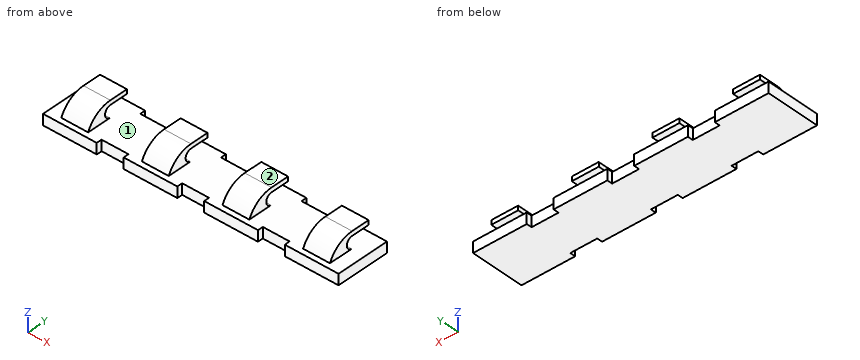
```python
from build123d import *

# Parameters (mm, degrees)
F0_W        = 5
F0_H        = 8
F1_DEPTH    = 2
F2_DEPTH    = 5
F3_T1_DEPTH = 27.9128784748
F3_T3_DEPTH = 27.9128784748
F3_T5_DEPTH = 27.9128784748
F3_T7_DEPTH = 27.9128784748
F5_DEPTH    = 65


# Not quite as in the source:
# - a fillet or chamfer that OpenCascade refuses, or shapes differently, is made with other operations: its cross-section is extruded or revolved along the edge and cut away or added


with BuildPart() as f1:
    # F0 (on Top) → F1 (new body)
    with BuildSketch(Plane.XY):
        Polygon((-17.5, 5), (-27.5, 5), (-27.5, -5), (-17.5, -5), (-17.5, -4), (-17.5, 4), align=None)
        with Locations((-22.5, 0)):
            Rectangle(F0_W, F0_H, mode=Mode.SUBTRACT)
        with Locations((-15, 0)):
            Rectangle(F0_W, F0_H)
        Polygon((-12.5, 5), (-12.5, 4), (-12.5, -4), (-12.5, -5), (-2.5, -5), (-2.5, -4), (-2.5, 4), (-2.5, 5), align=None)
        with Locations((-7.5, 0)):
            Rectangle(F0_W, F0_H, mode=Mode.SUBTRACT)
        Rectangle(F0_W, F0_H)
        Polygon((2.5, 5), (2.5, 4), (2.5, -4), (2.5, -5), (12.5, -5), (12.5, -4), (12.5, 4), (12.5, 5), align=None)
        with Locations((7.5, 0)):
            Rectangle(F0_W, F0_H, mode=Mode.SUBTRACT)
        with Locations((15, 0)):
            Rectangle(F0_W, F0_H)
        Polygon((17.5, 5), (17.5, 4), (17.5, -4), (17.5, -5), (27.5, -5), (27.5, 5), align=None)
        with Locations((22.5, 0)):
            Rectangle(F0_W, F0_H, mode=Mode.SUBTRACT)
    extrude(amount=F1_DEPTH)

    # F0 (on Top) → F2 (join)
    with BuildSketch(Plane.XY):
        with Locations((-22.5, 0)):
            Rectangle(F0_W, F0_H)
        with Locations((-7.5, 0)):
            Rectangle(F0_W, F0_H)
        with Locations((7.5, 0)):
            Rectangle(F0_W, F0_H)
        with Locations((22.5, 0)):
            Rectangle(F0_W, F0_H)
    extrude(amount=F2_DEPTH)

    # F3: fillet of radius 5 on 4 edges, made by hand

    # F3_s2 → F3_t1 (cut)
    with BuildSketch(Plane.YZ.offset(-36.4564392374)):
        with BuildLine():
            ThreePointArc((-4, 2), (-2.1560370926, 4.1833001327), (0.582575695, 5))
            Line((0.582575695, 5), (0.582575695, 5.1))
            Line((0.582575695, 5.1), (-4, 5.1))
            Line((-4, 5.1), (-4.1, 5))
            ThreePointArc((-4.1, 5), (-4.1, 3.5), (-4.0916515139, 2.04))
            Line((-4.0916515139, 2.04), (-4, 2))
        make_face()
    extrude(amount=F3_T1_DEPTH, mode=Mode.SUBTRACT)

    # F3_s4 → F3_t3 (cut)
    with BuildSketch(Plane.YZ.offset(-21.4564392374)):
        with BuildLine():
            ThreePointArc((-4, 2), (-2.1560370926, 4.1833001327), (0.582575695, 5))
            Line((0.582575695, 5), (0.582575695, 5.1))
            Line((0.582575695, 5.1), (-4, 5.1))
            Line((-4, 5.1), (-4.1, 5))
            ThreePointArc((-4.1, 5), (-4.1, 3.5), (-4.0916515139, 2.04))
            Line((-4.0916515139, 2.04), (-4, 2))
        make_face()
    extrude(amount=F3_T3_DEPTH, mode=Mode.SUBTRACT)

    # F3_s6 → F3_t5 (cut)
    with BuildSketch(Plane.YZ.offset(-6.4564392374)):
        with BuildLine():
            ThreePointArc((-4, 2), (-2.1560370926, 4.1833001327), (0.582575695, 5))
            Line((0.582575695, 5), (0.582575695, 5.1))
            Line((0.582575695, 5.1), (-4, 5.1))
            Line((-4, 5.1), (-4.1, 5))
            ThreePointArc((-4.1, 5), (-4.1, 3.5), (-4.0916515139, 2.04))
            Line((-4.0916515139, 2.04), (-4, 2))
        make_face()
    extrude(amount=F3_T5_DEPTH, mode=Mode.SUBTRACT)

    # F3_s8 → F3_t7 (cut)
    with BuildSketch(Plane.YZ.offset(8.5435607626)):
        with BuildLine():
            ThreePointArc((-4, 2), (-2.1560370926, 4.1833001327), (0.582575695, 5))
            Line((0.582575695, 5), (0.582575695, 5.1))
            Line((0.582575695, 5.1), (-4, 5.1))
            Line((-4, 5.1), (-4.1, 5))
            ThreePointArc((-4.1, 5), (-4.1, 3.5), (-4.0916515139, 2.04))
            Line((-4.0916515139, 2.04), (-4, 2))
        make_face()
    extrude(amount=F3_T7_DEPTH, mode=Mode.SUBTRACT)

    # F4 (on face) → F5 (cut)
    with BuildSketch(Plane(origin=(-25, 0, 0), x_dir=(0, -1, 0), z_dir=(-1, 0, 0))):
        with BuildLine():
            Line((-0.582575695, 4.1804881766), (-4, 4.1804881766))
            Line((-4, 4.1804881766), (-4, 2))
            Line((-4, 2), (-0.4667459871, 2))
            ThreePointArc((-0.4667459871, 2), (0.5092055571, 3.1451641031), (-0.582575695, 4.1804881766))
        make_face()
    extrude(amount=-F5_DEPTH, mode=Mode.SUBTRACT)


solid = f1.part
```
Here's how the part is built. I have some questions about the finished solid (model axes, mm). Face numbers are marked on the shaded views. Give positions to 0.01 mm unless a question says otherwise; leave off trailing zeros. Loops run counter-clockwise (first coordinate to the right, second up) from the corner with the lowest first, then second, coordinate; pieces in that order, holes last. Notation, with made-up numbers: M 55,41 L 62,41 A30 ccw 62,75 Z; hole C 8,-40 d6. An arc over 180 degrees is marked long. Return JSON: item names as keys, results as strings.
Item 1: I'm going to push flat-ended pins straight in: pin 1 Ø1.5 at (x, y) = (22, -2) entering from +Z; pin 2 Ø6 at (x, y) = (0.5, 2.5) entering from +Z; pin 3 Ø2.5 at (y, z) = (1, 4) entering from -X. Where does each tip first touch, or does it pass through?
A:
{"pin 1": "stops at z = 4.65", "pin 2": "stops at z = 2", "pin 3": "stops at x = -25"}
Item 2: Imagine slicing it at D-D on y = -3.5. List the corners of the cut face in (x, z) for me, then the cut area to 3 significant figures.
A:
{"outline": "M -27.5,0 L 27.5,0 L 27.5,2 L 25,2 L 25,2.89 L 20,2.89 L 20,2 L 10,2 L 10,2.89 L 5,2.89 L 5,2 L -5,2 L -5,2.89 L -10,2.89 L -10,2 L -20,2 L -20,2.89 L -25,2.89 L -25,2 L -27.5,2 Z", "area": "128 mm^2"}
Item 3: Imagine slicing it at B-B on z = 3.3. List the corners of the cut face in (x, y) for me, then the cut area to 3 significant figures.
A:
{"outline": "M -25,-3.17 L -20,-3.17 L -20,-0.49 L -25,-0.49 Z; M -10,-3.17 L -5,-3.17 L -5,-0.49 L -10,-0.49 Z; M 5,-3.17 L 10,-3.17 L 10,-0.49 L 5,-0.49 Z; M 20,-3.17 L 25,-3.17 L 25,-0.49 L 20,-0.49 Z", "area": "53.7 mm^2"}
Item 4: Please list where these lines run through material, in increasing order: line 1 (X direction, y = -4.25, z = 1.05); line 2 (X direction, y = -1.5, z = 3.65); line 3 (Z direction, x = 7.5, y = 1.5).
A:
{"line 1": "x = -27.5 to -17.5, -12.5 to -2.5, 2.5 to 12.5, 17.5 to 27.5", "line 2": "x = -25 to -20, -10 to -5, 5 to 10, 20 to 25", "line 3": "z = 0 to 2, 4.18 to 5"}
Item 5: Imagine slicing it at C-C on x = 12. List the corners of the cut face in (y, z) for me, then the cut area to 3 significant figures.
A:
{"outline": "M -5,0 L 5,0 L 5,2 L -5,2 Z", "area": "20.0 mm^2"}
Item 6: Imagine slicing it at A-A on y = 3. List the corners of the cut face in (x, z) for me.
A:
{"outline": "M -27.5,0 L 27.5,0 L 27.5,2 L -27.5,2 Z; M -25,4.18 L -20,4.18 L -20,5 L -25,5 Z; M -10,4.18 L -5,4.18 L -5,5 L -10,5 Z; M 5,4.18 L 10,4.18 L 10,5 L 5,5 Z; M 20,4.18 L 25,4.18 L 25,5 L 20,5 Z"}
Item 7: Thinking about a two-plate mould opening in X: for the marked faces 1 and 2, which applies, released by +X, released by -X, zero draft, split by the parting line, or undercut?
A:
{"face 1": "undercut", "face 2": "zero draft"}
